Work out the finished part from the listing and answer in its coordinate system (mm). A direction names the side the tool comes from. Coordinates: 2 decimals unless noted, no trailing zeros. Use CSV: the item, a comma, the result in double quotes.
from build123d import *

# Parameters (mm, degrees)
SKETCH1_W                                       = 101.6
SKETCH1_H                                       = 31.75
BOSS_EXTRUDE1_DEPTH                             = 6.35
M5X0_8_TAPPED_HOLE1_D                           = 4.2
M5X0_8_TAPPED_HOLE1_DEPTH                       = 10.9301927
M5X0_8_TAPPED_HOLE1_TIP                         = 1.2618073
CSK_FOR_M5_FLAT_HEAD_MACHINE_SCREW1_D           = 5.5
CSK_FOR_M5_FLAT_HEAD_MACHINE_SCREW1_DEPTH       = 10.539633298
CSK_FOR_M5_FLAT_HEAD_MACHINE_SCREW1_CSINK_D     = 10.4
CSK_FOR_M5_FLAT_HEAD_MACHINE_SCREW1_CSINK_ANGLE = 90
CSK_FOR_M5_FLAT_HEAD_MACHINE_SCREW1_TIP         = 1.652366702


with BuildPart() as part:
    # Sketch1 → Boss-Extrude1 (new, symmetric)
    with BuildSketch(Plane(origin=(0, 0, 0), x_dir=(1, 0, 0), z_dir=(0, 1, 0))):
        Rectangle(SKETCH1_W, SKETCH1_H)
    extrude(amount=BOSS_EXTRUDE1_DEPTH, both=True)

    # M5x0.8 Tapped Hole1
    with Locations(Plane(origin=(50.8, 0, 0), x_dir=(0, 0, -1), z_dir=(1, 0, 0))):
        with Locations((-9.525, 0), (9.525, 0)):
            Hole(M5X0_8_TAPPED_HOLE1_D / 2, depth=M5X0_8_TAPPED_HOLE1_DEPTH)
            with Locations((0, 0, -(M5X0_8_TAPPED_HOLE1_DEPTH + M5X0_8_TAPPED_HOLE1_TIP / 2))):  # 118° drill point
                Cone(0, M5X0_8_TAPPED_HOLE1_D / 2, M5X0_8_TAPPED_HOLE1_TIP, mode=Mode.SUBTRACT)

    # CSK for M5 Flat Head Machine Screw1
    with Locations(Plane(origin=(0, 6.35, 0), x_dir=(1, 0, 0), z_dir=(0, 1, 0))):
        with Locations((-44.45, -9.525), (-44.45, 9.525)):
            CounterSinkHole(CSK_FOR_M5_FLAT_HEAD_MACHINE_SCREW1_D / 2, CSK_FOR_M5_FLAT_HEAD_MACHINE_SCREW1_CSINK_D / 2, depth=CSK_FOR_M5_FLAT_HEAD_MACHINE_SCREW1_DEPTH, counter_sink_angle=CSK_FOR_M5_FLAT_HEAD_MACHINE_SCREW1_CSINK_ANGLE)
            with Locations((0, 0, -(CSK_FOR_M5_FLAT_HEAD_MACHINE_SCREW1_DEPTH + CSK_FOR_M5_FLAT_HEAD_MACHINE_SCREW1_TIP / 2))):  # 118° drill point
                Cone(0, CSK_FOR_M5_FLAT_HEAD_MACHINE_SCREW1_D / 2, CSK_FOR_M5_FLAT_HEAD_MACHINE_SCREW1_TIP, mode=Mode.SUBTRACT)


solid = part.part
Item 1: Given pin 1 (2.5 mm diameter, centred on y = 0, z = 9.525, fed in from +X), flat-ended and moving along its own axis, determine where the tip first touches the part or whether it passes through.
Answer:
pin 1,"stops at x = 39.36"
Item 2: For a pull along Z with two mould halves and no side action, classify faces 1 (the face through (-50.8, 0, 0)), 2 (the face through (-1, 0, 15.875)), 3 (the face through (-47.1, 4.02, -8.43)) as released by +Z, released by -Z, zero draft, split by the parting line, or undercut.
Answer:
face 1,"zero draft"
face 2,"released by +Z"
face 3,"undercut"
Item 3: A tool of negligible diameter and unlimited length cuts with its end or side. For faces 4 (the face through (-47, -0.2, -8.5)), 5 (the face through (45.26, 0.63, -7.52)), 6 (the face through (-1, 6.35, 0)), from which of +Z, -Z, +X, -X, +Y, -Y can it reach the whole face along a straight path? Write none if from no direction.
Answer:
face 4,"+Y"
face 5,"+X"
face 6,"+Z, -Z, +X, -X, +Y"
Item 4: Consider probe 1 along Z at (x, y) = (47.25, 0) (3 decimals); probe 2 along X at (y, z) = (-1, -12); probe 3 along Z at (x, y) = (-45.5, 5) (3 decimals). Determine where each line is inside the solid, lowest interval first.
Answer:
probe 1,"z = -15.875 to -11.625, -7.425 to 7.425, 11.625 to 15.875"
probe 2,"x = -50.8 to -45.65, -43.25 to 50.8"
probe 3,"z = -15.875 to -13.229, -5.821 to 5.821, 13.229 to 15.875"
